Read the model definition and answer for the solid it produces. Units are mm, in the model's axes. Face numbers are marked on the shaded views. A direction names the side the tool comes from. Give positions to 0.01 mm unless a question says otherwise; leave off trailing zeros. Order: outer loops, then holes, each group sorted by start corner. A loop starts at its lowest first (then second) coordinate and runs counter-clockwise, first axis right, second up.
Item 1: Find the intervals of material crossed by line 1 along X through (y, z) = (5, 0); line 2 along X through (y, z) = (-6, 0); line 3 along Z through (x, y) = (-17, -4.75), in increasing order.
Item 2: A cutting plane is placed at D-D (x = -144.5). Write down the section's boundary in (y, z), plus the area to 3 significant figures.
Item 3: A cutting plane is placed at C-C (x = -17). Write down the section's boundary in (y, z).
Item 4: Which of the six approach directions +Z, -Z, +X, -X, +Y, -Y give full straight-line access (tool end or side, diameter ignored) to the marked faces 1, 2 and 3?
Item 5: A cutting plane is placed at B-B (z = 7.5). Write down the section's boundary in (x, y), plus the area to 3 significant figures.
Item 6: A cutting plane is placed at A-A (y = 4.75). Write down the section's boundary in (x, z), plus the area to 3 significant figures.
Item 7: Given pin 1 Ø5.5 at (x, z) = (-150.5, 0) entering from -Y; pin 2 Ø4 at (x, z) = (-46.5, 4) entering from +Y; pin 3 Ø12 at (x, z) = (-104, 7.5) entering from +Y; pin 4 Ø6.5 at (x, z) = (-17, 0) entering from +Y, each flat-ended and moving along its own axis, determine where each tip first touches the part or whether it passes through.
Autodesk Inventor part; units mm, degrees
ref_plane "作業平面1" through (0, 9, 0) normal (0, 1, 0) x (-1, 0, 0)
ref_plane "YZ Plane" through (0, 0, 0) normal (1, 0, 0) x (0, 1, 0)
ref_plane "XY Plane" through (0, 0, 0) normal (0, 0, 1) x (1, 0, 0)
sketch "スケッチ1" plane through (0, 0, 0) normal (0, 1, 0) x (-1, 0, 0)
  line L0 (204, 0) -> (-34, 0)
  line L1 (0, -13.2) -> (0, 2.2)
  line L2 (170, 0) -> (170, -9)
  line L3 (118, -11) -> (98, -11)
  line L4 (98, -11) -> (98, -10)
  line L5 (98, -10) -> (0, -10)
  line L6 (0, -10) -> (0, 0)
  line L7 (170, 0) -> (0, 0)
  line L8 (170, -9) -> (141, -9)
  line L9 (141, -9) -> (141, -10)
  line L10 (141, -10) -> (118, -10)
  line L11 (118, -10) -> (118, -11)
  dimension "d1" = 11
  dimension "d2" = 10
  dimension "d3" = 9
  dimension "d4" = 10
  dimension "d6" = 29
  dimension "d8" = 23
  dimension "d9" = 20
  dimension "d10" = 170
revolve "回転1" add sketch "スケッチ1" angle 360 about axis through (-170, 0, 0) along (1, 0, 0)
sketch "スケッチ2" plane through (0, 0, 0) normal (0, 1, 0) x (-1, 0, 0)
  circle A0 centre (17, 0) radius 4
  line L0 (0, 10) -> (0, -10)
  point P0 (0, 0)
  dimension "d12" = 8
  dimension "d13" = 17
extrude "押し出し2" cut sketch "スケッチ2" along normal through all both and the other way through all
ref_plane "作業平面1" through (0, 9, 0) normal (0, 1, 0) x (-1, 0, 0)
sketch "スケッチ3" plane through (0, 9, 0) normal (0, 1, 0) x (-1, 0, 0)
  line L0 (170, 9) -> (170, -9)
  point P0 (0, 0)
  point P1 (150.5, 0)
  dimension "d19" = 19.5
hole "穴1" at (-150.5, 9, 0) direction (0, -1, 0) diameter 6 depth 8 tip angle 118
properties part number "Shaft_main" material "アルミニウム 6061"
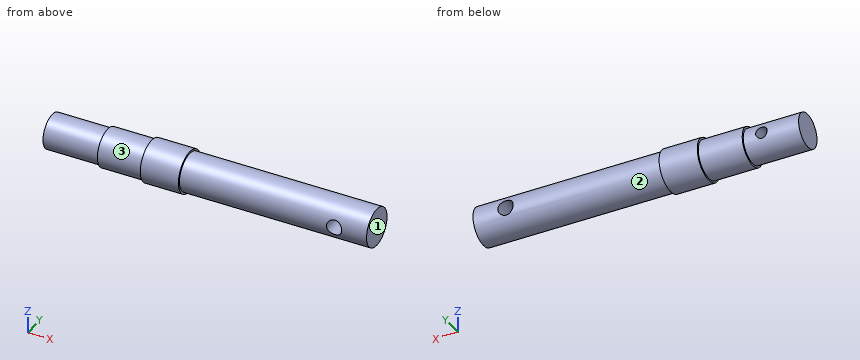
Response values:
1. line 1: x = -170 to -153.5, -147.5 to -21, -13 to 0
1. line 2: x = -170 to -21, -13 to 0
1. line 3: z = -8.8 to -4, 4 to 8.8
2. outline: circle Ø18 at (0, 0)
2. area: 254 mm2
3. outline: (-9.17, -4) arc R10 ccw to (9.17, -4) - close; (-9.17, 4) - (9.17, 4) arc R10 ccw to start
4. face 1: +Z, -Z, +X, +Y, -Y
4. face 2: +X
4. face 3: -X
5. outline: (-170, -4.97) - (-141, -4.97) - (-141, -6.61) - (-118, -6.61) - (-118, -8.05) - (-98, -8.05) - (-98, -6.61) - (0, -6.61) - (0, 6.61) - (-98, 6.61) - (-98, 8.05) - (-118, 8.05) - (-118, 6.61) - (-141, 6.61) - (-141, 4.97) - (-170, 4.97) - close
5. area: 2,210 mm2
6. outline: (-170, -7.64) - (-141, -7.64) - (-141, -8.8) - (-118, -8.8) - (-118, -9.92) - (-98, -9.92) - (-98, -8.8) - (0, -8.8) - (0, 8.8) - (-98, 8.8) - (-98, 9.92) - (-118, 9.92) - (-118, 8.8) - (-141, 8.8) - (-141, 7.64) - (-170, 7.64) - close; hole circle Ø6 at (-150.5, 0); hole circle Ø8 at (-17, 0)
6. area: 2,890 mm2
7. pin 1: stops at y = -9
7. pin 2: stops at y = 9.8
7. pin 3: stops at y = 10.9
7. pin 4: passes through
